from build123d import *

# Parameters (mm, degrees)
SKETCH1_W              = 54
SKETCH1_H              = 39.25
BOSS_EXTRUDE1_DEPTH    = 15.5
FILLET1_R              = 2
FILLET2_R              = 2
M3_A_START             = -2.329776532
M3_A_BLANK_DEPTH       = 8
M3_A_START_2           = -3.329776532
M3_A_BLANK_2_DEPTH     = 1
M3_A_START_3           = -9.329776532
M3_A_BLANK_3_OUTLINE_R = 2.5
M3_A_BLANK_3_DEPTH     = 6
BODY_MOVE_COPY6_ANGLE  = 90
CUT_EXTRUDE1_DEPTH     = 13.5
SKETCH4_R              = 4.500854338
CUT_EXTRUDE3_DEPTH     = 5
CUT_EXTRUDE4_DEPTH     = 1


with BuildPart() as part:
    # Sketch1 → Boss-Extrude1 (new body)
    with BuildSketch(Plane(origin=(0, 0, 0), x_dir=(1, 0, 0), z_dir=(0, 1, 0))):
        with Locations((27, 19.625)):
            Rectangle(SKETCH1_W, SKETCH1_H)
    extrude(amount=BOSS_EXTRUDE1_DEPTH)

    # Fillet1
    fillet1_edges = [part.edges().sort_by_distance(p)[0] for p in [
        (0, 7.75, 0),
    ]]
    fillet(fillet1_edges, radius=FILLET1_R)

    # Fillet2
    fillet2_edges = [part.edges().sort_by_distance(p)[0] for p in [
        (0, 7.75, -39.25),
        (54, 7.75, -39.25),
        (54, 7.75, 0),
    ]]
    fillet(fillet2_edges, radius=FILLET2_R)


with BuildPart() as body_2:
    # M3-A Blank: read off the stored shape, not the designer's step
    # M3-A Blank outline → M3-A Blank (new body)
    with BuildSketch(Plane(origin=(0, 0, 0), x_dir=(1, 0, 0), z_dir=(0, 1, 0)).offset(M3_A_START)):
        with BuildLine():
            Line((-21.79493826, 68.00205199), (-26.79493826, 68.00205199))
            Line((-26.79493826, 68.00205199), (-26.79493826, 76.75205199))
            Line((-26.79493826, 76.75205199), (-30.19493826, 76.75205199))
            Line((-30.19493826, 76.75205199), (-35.227586031, 68.720149487))
            Line((-35.227586031, 68.720149487), (-35.685099465, 57.485652948))
            Line((-35.685099465, 57.485652948), (-41.581939277, 52.808848959))
            Line((-41.581939277, 52.808848959), (-41.581939277, 43.861919588))
            Line((-41.581939277, 43.861919588), (-30.381939277, 42.692718591))
            ThreePointArc((-30.381939277, 42.692718591), (-24.381939277, 38.532817401), (-18.381939277, 42.692718591))
            Line((-18.381939277, 42.692718591), (-7.181939277, 43.861919588))
            Line((-7.181939277, 43.861919588), (-7.181939277, 52.808848959))
            Line((-7.181939277, 52.808848959), (-13.057281533, 57.485652948))
            Line((-13.057281533, 57.485652948), (-13.463960141, 68.720149487))
            Line((-13.463960141, 68.720149487), (-18.39493826, 76.75205199))
            Line((-18.39493826, 76.75205199), (-21.79493826, 76.75205199))
            Line((-21.79493826, 76.75205199), (-21.79493826, 68.00205199))
        make_face()
    extrude(amount=M3_A_BLANK_DEPTH)

    # M3-A Blank 2 outline → M3-A Blank 2 (add)
    with BuildSketch(Plane(origin=(0, 0, 0), x_dir=(1, 0, 0), z_dir=(0, 1, 0)).offset(M3_A_START_2)):
        with BuildLine():
            Line((-30.381939277, 58.496246856), (-30.381939277, 42.692718591))
            ThreePointArc((-30.381939277, 42.692718591), (-24.381939277, 38.532817401), (-18.381939277, 42.692718591))
            Line((-18.381939277, 42.692718591), (-18.381939277, 58.496246856))
            Line((-18.381939277, 58.496246856), (-21.79493826, 68.00205199))
            Line((-21.79493826, 68.00205199), (-26.79493826, 68.00205199))
            Line((-26.79493826, 68.00205199), (-30.381939277, 58.496246856))
        make_face()
    extrude(amount=M3_A_BLANK_2_DEPTH)

    # M3-A Blank 3 outline → M3-A Blank 3 (add)
    with BuildSketch(Plane(origin=(0, 0, 0), x_dir=(1, 0, 0), z_dir=(0, 1, 0)).offset(M3_A_START_3)):
        with Locations((-24.335480832, 54.269355582)):
            Circle(M3_A_BLANK_3_OUTLINE_R)
    extrude(amount=M3_A_BLANK_3_DEPTH)


with BuildPart() as body_2_1:
    # Body-Move/Copy4: moved
    add(body_2.part.moved(Location((42.5, 8.919688157, 37.96700657))))


with BuildPart() as body_2_2:
    # Body-Move/Copy5: moved
    add(body_2_1.part.moved(Location((8.915108254, 0, 0))))


with BuildPart() as body_2_3:
    # Body-Move/Copy6: moved
    add(body_2_2.part.rotate(Axis((27.033168977, 0, -19.675428126), (0, 1, 0)), BODY_MOVE_COPY6_ANGLE))


with BuildPart() as body_2_4:
    # Body-Move/Copy7: moved
    add(body_2_3.part.moved(Location((0, 1.103676274, 0))))


with BuildPart() as body_2_5:
    # Body-Move/Copy8: moved
    add(body_2_4.part.moved(Location((0, 0.5, 0))))


with BuildPart() as part_1:
    add(part.part)

    # Intersect1: read off the stored shape, not the designer's step
    # Intersect1: cut body 2
    add(body_2_5.part, mode=Mode.SUBTRACT)

    # Sketch3 → Cut-Extrude1 (cut)
    with BuildSketch(Plane(origin=(0, 0, 0), x_dir=(-1, 0, 0), z_dir=(0, -1, 0))):
        Polygon((-5.923551682, 12.755419679), (-16.048628272, 6.41122612), (-26.192603819, 6.41122612), (-29.691162465, 2), (-2, 2), (-2, 14.017695962), (-5.923551682, 14.017695962), align=None)
        Polygon((-2, 37.25), (-29.60864948, 37.25), (-26.198159594, 32.965493874), (-15.357384062, 32.57306761), (-5.923551682, 26.781411023), (-5.923551682, 25.507817982), (-2, 25.507817982), align=None)
        Polygon((-5.923551682, 20.262429143), (-14.673551682, 20.262429143), (-14.673551682, 19.262429143), (-5.923551682, 19.262429143), (-5.923551682, 16.008924411), (-2, 16.008924411), (-2, 23.521920083), (-5.923551682, 23.521920083), align=None)
        with BuildLine():
            Line((-42.774921098, 2), (-52, 2))
            Line((-52, 2), (-52, 18.627764364))
            Line((-52, 18.627764364), (-48.077251764, 18.627764364))
            ThreePointArc((-48.077251764, 18.627764364), (-46.712904885, 14.985289801), (-43.85505184, 12.346778986))
            Line((-43.85505184, 12.346778986), (-42.774921098, 2))
        make_face()
        with BuildLine():
            Line((-52, 37.25), (-42.78544978, 37.25))
            Line((-42.78544978, 37.25), (-43.85505184, 27.004077266))
            ThreePointArc((-43.85505184, 27.004077266), (-46.741831066, 24.322246322), (-48.089593706, 20.619646239))
            Line((-48.089593706, 20.619646239), (-52, 20.619646239))
            Line((-52, 20.619646239), (-52, 37.25))
        make_face()
    extrude(amount=-CUT_EXTRUDE1_DEPTH, mode=Mode.SUBTRACT)

    # Sketch4 → Cut-Extrude3 (cut)
    with BuildSketch(Plane.XZ):
        with BuildLine():
            Line((5.923551682, -14.017695962), (5.923551682, -12.755419679))
            Line((5.923551682, -12.755419679), (16.048628272, -6.41122612))
            Line((16.048628272, -6.41122612), (26.192603819, -6.41122612))
            Line((26.192603819, -6.41122612), (29.691162465, -2))
            Line((29.691162465, -2), (42.774921098, -2))
            Line((42.774921098, -2), (43.85505184, -12.346778986))
            ThreePointArc((43.85505184, -12.346778986), (48.142786272, -19.675428126), (43.85505184, -27.004077266))
            Line((43.85505184, -27.004077266), (42.78544978, -37.25))
            Line((42.78544978, -37.25), (29.60864948, -37.25))
            Line((29.60864948, -37.25), (26.198159594, -32.965493874))
            Line((26.198159594, -32.965493874), (15.357384062, -32.57306761))
            Line((15.357384062, -32.57306761), (5.923551682, -26.781411023))
            Line((5.923551682, -26.781411023), (5.923551682, -25.507817982))
            Line((5.923551682, -25.507817982), (5.923551682, -23.521920083))
            Line((5.923551682, -23.521920083), (5.923551682, -20.262429143))
            Line((5.923551682, -20.262429143), (5.923551682, -19.262429143))
            Line((5.923551682, -19.262429143), (5.923551682, -16.008924411))
            Line((5.923551682, -16.008924411), (5.923551682, -14.017695962))
        make_face()
        with Locations(Location((30.40624809, -19.721886571, 0), (0, 0, 270))):
            Circle(SKETCH4_R, mode=Mode.SUBTRACT)
    extrude(amount=-CUT_EXTRUDE3_DEPTH, mode=Mode.SUBTRACT)

    # Sketch5 → Cut-Extrude4 (cut)
    with BuildSketch(Plane.XZ.offset(-5)):
        Polygon((43.85505184, -12.346778986), (42.774921098, -2), (29.691162465, -2), (26.192603819, -6.41122612), (16.048628272, -6.41122612), (5.923551682, -12.755419679), (5.923551682, -19.262429143), (14.673551682, -19.262429143), (14.673551682, -17.262429143), (24.035435238, -12.346778986), align=None)
        Polygon((14.673551682, -20.262429143), (5.923551682, -20.262429143), (5.923551682, -26.781411023), (15.357384062, -32.57306761), (26.198159594, -32.965493874), (29.60864948, -37.25), (42.78544978, -37.25), (43.85505184, -27.004077266), (23.961363008, -27.004077266), (14.673551682, -22.262429143), align=None)
    extrude(amount=-CUT_EXTRUDE4_DEPTH, mode=Mode.SUBTRACT)


solid = part_1.part
Verification items for the finished model (mm, model axes). A direction names the side the tool comes from. Coordinates: 2 decimals unless noted, no trailing zeros. Order: outer loops, then holes, each group sorted by start corner. A loop starts at its lowest first (then second) coordinate and runs counter-clockwise, first axis right, second up.
1. Sectioned sample at A-A, the plane x = 4. Record the cut outline in (y, z).
Results found:
outline: (0, -39.25) - (15.5, -39.25) - (15.5, 0) - (0, 0) - (0, -2) - (13.5, -2) - (13.5, -14.02) - (0, -14.02) - (0, -16.01) - (13.5, -16.01) - (13.5, -23.52) - (0, -23.52) - (0, -25.51) - (13.5, -25.51) - (13.5, -37.25) - (0, -37.25) - close
2. Scan lines: line 1 (Z direction, x = 5, y = 2.5); line 2 (Z direction, x = 16, y = 13.75); line 3 (X direction, y = 4.25, z = -13.5). Record each from-to range of solid material in increasing order.
Results found:
line 1: z = -39.25 to -37.25, -25.51 to -23.52, -16.01 to -14.02, -2 to 0
line 2: z = -39.25 to -30.6, -22.26 to -17.26, -8.83 to 0
line 3: x = 0 to 2, 52 to 54
3. Set-up check for faces 1 (the face through (21.494, 11.796, -8.604)), 2 (the face through (27, 7, -2)): record each of +Z, -Z, +X, -X, +Y, -Y from which the full face is reachable in a straight line by a thin tool's end or side.
Results found:
face 1: +Y
face 2: -Y
4. Go/stop test with flat-tipped pins: pin 1 Ø9.5 at (x, z) = (9.5, -7) entering from -Y; pin 2 Ø12 at (x, z) = (14.5, -29) entering from +Y; pin 3 Ø4.5 at (x, z) = (30.41, -19.72) entering from +Y. Record where each tip stops, or that it passes through.
Results found:
pin 1: stops at y = 6
pin 2: stops at y = 15.5
pin 3: stops at y = 1.19
5. Sectioned sample at D-D, the plane y = 11. Give the number of separate pieces and of enclosed holes in the cut face, and give its area (3 significant figures).
Results found:
separate pieces: 1
enclosed holes: 6
area: 637 mm2
6. Release check for a two-part mould opening along X. For faces 3 (the face through (27, 0, -39)), 4 (the face through (0, 8, -19)), 5 (the face through (32.847, 4.152, -19.18)) record: +X half, -X half, draft (parallel to the pull), parting line (faces both ways), or undercut.
Results found:
face 3: draft
face 4: -X half
face 5: undercut
7. Sectioned sample at B-B, the plane y = 3.25. Record the cut outline in (x, z), and give its area (3 significant figures).
Results found:
outline: (0, -37.25) arc R2 ccw to (2, -39.25) - (52, -39.25) arc R2 ccw to (54, -37.25) - (54, -2) arc R2 ccw to (52, 0) - (2, 0) arc R2 ccw to (0, -2) - close; circle Ø9 at (30.41, -19.72); hole (2, -37.25) - (52, -37.25) - (52, -20.62) - (48.09, -20.62) arc R8.41 ccw to (48.08, -18.63) - (52, -18.63) - (52, -2) - (2, -2) - (2, -14.02) - (5.92, -14.02) - (5.92, -16.01) - (2, -16.01) - (2, -23.52) - (5.92, -23.52) - (5.92, -25.51) - (2, -25.51) - close; hole circle Ø5 at (30.41, -19.72)
area: 421 mm2
8. Sectioned sample at C-C, the plane z = -29.5. Record the cut outline in (x, y).
Results found:
outline: (0, 0) - (2, 0) - (2, 13.5) - (10.35, 13.5) - (10.35, 6) - (43.59, 6) - (43.59, 13.5) - (52, 13.5) - (52, 0) - (54, 0) - (54, 15.5) - (41.58, 15.5) - (41.58, 8.19) - (14.17, 8.19) - (14.17, 15.5) - (0, 15.5) - close
